```python
from build123d import *

# Parameters (mm, degrees)
F1_DEPTH = 100
F2_DEPTH = 9


with BuildPart() as f1:
    # F0 (on Top) → F1 (new body)
    with BuildSketch(Plane.XY):
        with BuildLine():
            ThreePointArc((150, 77.5), (147.071068, 84.571068), (140, 87.5))
            Line((140, 87.5), (-140, 87.5))
            ThreePointArc((-140, 87.5), (-147.071068, 84.571068), (-150, 77.5))
            Line((-150, 77.5), (-150, -77.5))
            ThreePointArc((-150, -77.5), (-147.071068, -84.571068), (-140, -87.5))
            Line((-140, -87.5), (140, -87.5))
            ThreePointArc((140, -87.5), (147.071068, -84.571068), (150, -77.5))
            Line((150, -77.5), (150, 77.5))
        make_face()
        with BuildLine():
            ThreePointArc((140, 82.5), (143.535534, 81.035534), (145, 77.5))
            Line((145, 77.5), (145, -77.5))
            ThreePointArc((145, -77.5), (143.535534, -81.035534), (140, -82.5))
            Line((140, -82.5), (-140, -82.5))
            ThreePointArc((-140, -82.5), (-143.535534, -81.035534), (-145, -77.5))
            Line((-145, -77.5), (-145, 77.5))
            ThreePointArc((-145, 77.5), (-143.535534, 81.035534), (-140, 82.5))
            Line((-140, 82.5), (140, 82.5))
        make_face(mode=Mode.SUBTRACT)
    extrude(amount=-F1_DEPTH)

    # F0 (on Top) → F2 (join)
    with BuildSketch(Plane.XY):
        with BuildLine():
            Line((145, -77.5), (145, 77.5))
            ThreePointArc((145, 77.5), (143.535534, 81.035534), (140, 82.5))
            Line((140, 82.5), (-140, 82.5))
            ThreePointArc((-140, 82.5), (-143.535534, 81.035534), (-145, 77.5))
            Line((-145, 77.5), (-145, -77.5))
            ThreePointArc((-145, -77.5), (-143.535534, -81.035534), (-140, -82.5))
            Line((-140, -82.5), (140, -82.5))
            ThreePointArc((140, -82.5), (143.535534, -81.035534), (145, -77.5))
        make_face()
    extrude(amount=-F2_DEPTH)


solid = f1.part
```
Check sheet for the modelled part. Datum: model origin and axes. Units: mm. A direction names the side the tool comes from. Coordinates: 2 decimals unless noted, no trailing zeros. Write each loop counter-clockwise with the first axis right and the second up, starting at its lowest first coordinate (ties: lowest second). Pieces come first, ordered by that corner, then holes. Notation, with made-up numbers: M -33.5,62 L 1.5,62 A14 ccw 1.5,74 Z; hole C 25.25,-31 d9. An arc over 180 degrees is marked long. Write item = value, one per line. Start each with the question number.
1. Sectioned sample at C-C (y = -64). Record the cut outline in (x, z), then the cut area to 3 significant figures.
2. Sectioned sample at A-A (z = -70.5). Record the cut outline in (x, y).
3. Go/stop test with a flat-tipped pin: pin 1 (1 mm diameter, centred on x = 70.5, y = -56, fed in from -Z). Record where the tip stops, or that it passes through.
4. Tool access check on faces 4 (the flat face through (150, -1, -49)), 5 (the flat face through (2, -82.5, -54)). Record the directions out of +Z, -Z, +X, -X, +Y, -Y that give a thin tool (end or side, any length) a straight path to the whole face; none if there is none.
5. Mould release check, pull along X, two halves, no side actions. Record for faces 1 (the flat face through (-2, 1, -9)), 2 (the flat face through (-150, 1, -49)), 3 (the flat face through (-2, -87.5, -49)): pulls with the +X half, pulls with the -X half, needs draft (parallel to the pull), parting line crosses it, or undercut.
6. Sectioned sample at B-B (x = 55.5). Record the cut outline in (y, z), then the cut area to 4 significant figures.
7. Thickness scan on probe 1 along Y at (x, z) = (-85.5, -43.5); probe 2 along X at (y, z) = (-12, -37); probe 3 along Z at (x, y) = (-125.5, 46). Record the ranges inside material, lowest first.
The answers:
q1.outline = M -150,-100 L -145,-100 L -145,-9 L 145,-9 L 145,-100 L 150,-100 L 150,0 L -150,0 Z
q1.area = 3,610 mm²
q2.outline = M -150,-77.5 A10 ccw -140,-87.5 L 140,-87.5 A10 ccw 150,-77.5 L 150,77.5 A10 ccw 140,87.5 L -140,87.5 A10 ccw -150,77.5 Z; hole M -145,-77.5 A5 ccw -140,-82.5 L 140,-82.5 A5 ccw 145,-77.5 L 145,77.5 A5 ccw 140,82.5 L -140,82.5 A5 ccw -145,77.5 Z
q3.pin_1 = -9
q4.face_4 = +Z, -Z, +X, +Y, -Y
q4.face_5 = -Z
q5.face_1 = undercut
q5.face_2 = pulls with the -X half
q5.face_3 = needs draft
q6.outline = M -87.5,-100 L -82.5,-100 L -82.5,-9 L 82.5,-9 L 82.5,-100 L 87.5,-100 L 87.5,0 L -87.5,0 Z
q6.area = 2,485 mm²
q7.probe_1 = -87.5 to -82.5, 82.5 to 87.5
q7.probe_2 = -150 to -145, 145 to 150
q7.probe_3 = -9 to 0
